Can you work these out from the model? Positions are in its coordinate system, mm. Face numbers are marked on the shaded views. A direction names the side the tool comes from. Round coordinates to 2 decimals unless told otherwise and drop trailing zeros. Write each loop counter-clockwise with the first axis right and the second up, starting at its lowest first coordinate (ties: lowest second). Pieces come first, ordered by that corner, then holes. Notation, with made-up numbers: M 54,73.25 L 62,73.25 A25 ccw 62,99.25 Z; hole C -9.75,22 d7. An arc over 180 degrees is marked long. Answer in a Markdown table with one row per item. Add a question column.
(1) Suppose I cut it at D-D, the plane z = 0.75. Write out the boundary of the cut face in (x, y).
(2) If I drill on probe 1 along X at (y, z) = (1, 5.5); probe 2 along Z at (x, y) = (-6, -5.75); probe 3 along Y at (x, z) = (-1.25, -2.5), over which ranges is the centre line in solid material (lowest first)?
(3) Suppose I cut it at A-A, the plane z = -5.5. Write out the boundary of the cut face in (x, y) (3 decimals), then the cut area to 3 significant figures.
(4) For the marked faces 1, 2 and 3, which set-ups out of +Z, -Z, +X, -X, +Y, -Y let a thin tool reach every point of the face, with its end or its side?
(5) I'm going to push flat-ended pins straight in: pin 1 (2.5 mm diameter, centred on x = -9, z = 5.5, fed in from +Y); pin 2 (1 mm diameter, centred on x = -4.5, y = -6.5, fed in from +Z); pin 3 (3 mm diameter, centred on x = 9, z = -5.5, fed in from -Y); pin 4 (0.9 mm diameter, centred on y = -2.5, z = -18, fed in from +X). Where does each tip first touch, or does it pass through?
(6) Suppose I cut it at B-B, the plane x = 9. Write out the boundary of the cut face in (y, z) (3 decimals).
(7) Suppose I cut it at C-C, the plane y = 1. Write out the boundary of the cut face in (x, z), then the cut area to 3 significant figures.
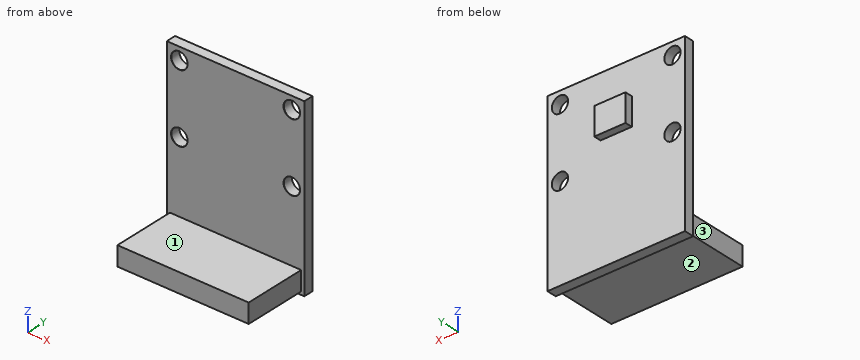
from build123d import *

# Parameters (mm, degrees)
SKETCH1_W                           = 22
SKETCH1_H                           = 28
BOSS_EXTRUDE1_DEPTH                 = 1.57
F_2_6_2_6_DIAMETER_HOLE1_AT_2_COUNT = 2
F_2_6_2_6_DIAMETER_HOLE1_AT_2_PITCH = 11
F_2_6_2_6_DIAMETER_HOLE1_AT_3_COUNT = 2
F_2_6_2_6_DIAMETER_HOLE1_AT_3_PITCH = 21.09502311
F_2_6_2_6_DIAMETER_HOLE1_AT_4_COUNT = 2
F_2_6_2_6_DIAMETER_HOLE1_AT_4_PITCH = 18
SKETCH5_W                           = 5
SKETCH5_H                           = 4.4
BOSS_EXTRUDE2_DEPTH                 = 1.2
SKETCH6_W                           = 21
SKETCH6_H                           = 3.08
BOSS_EXTRUDE3_DEPTH                 = 10


with BuildPart() as part:
    # Sketch1 → Boss-Extrude1 (new body)
    with BuildSketch(Plane(origin=(0, 0, 0), x_dir=(1, 0, 0), z_dir=(0, 1, 0))):
        with Locations((0, 6.5)):
            Rectangle(SKETCH1_W, SKETCH1_H)
    extrude(amount=BOSS_EXTRUDE1_DEPTH)

    # Sketch3 → Ø2.6 (2.6) Diameter Hole1 (revolve, cut)
    with BuildSketch(Plane(origin=(-9, 1.57, -5.5), x_dir=(0, 0, 1), z_dir=(1, 0, 0))):
        Polygon((0, 0), (0, 1.57), (1.325, 1.57), (1.3, 1.545), (1.3, 0), align=None)
    f_2_6_2_6_diameter_hole1 = revolve(axis=Axis((-9, 7.92, -5.5), (0, -1, 0)), mode=Mode.SUBTRACT)

    # Ø2.6 (2.6) Diameter Hole1 at 2: Ø2.6 (2.6) Diameter Hole1 ×2
    with Locations(*[(0, 0, i * F_2_6_2_6_DIAMETER_HOLE1_AT_2_PITCH) for i in range(1, F_2_6_2_6_DIAMETER_HOLE1_AT_2_COUNT)]):
        add(f_2_6_2_6_diameter_hole1, mode=Mode.SUBTRACT)

    # Ø2.6 (2.6) Diameter Hole1 at 3: Ø2.6 (2.6) Diameter Hole1 ×2
    with Locations(*[Vector(0.853281834, 0, 0.521450009) * (i * F_2_6_2_6_DIAMETER_HOLE1_AT_3_PITCH) for i in range(1, F_2_6_2_6_DIAMETER_HOLE1_AT_3_COUNT)]):
        add(f_2_6_2_6_diameter_hole1, mode=Mode.SUBTRACT)

    # Ø2.6 (2.6) Diameter Hole1 at 4: Ø2.6 (2.6) Diameter Hole1 ×2
    with Locations(*[(i * F_2_6_2_6_DIAMETER_HOLE1_AT_4_PITCH, 0, 0) for i in range(1, F_2_6_2_6_DIAMETER_HOLE1_AT_4_COUNT)]):
        add(f_2_6_2_6_diameter_hole1, mode=Mode.SUBTRACT)

    # Sketch5 → Boss-Extrude2 (add)
    with BuildSketch(Plane(origin=(0, 1.57, 0), x_dir=(1, 0, 0), z_dir=(0, 1, 0))):
        Rectangle(SKETCH5_W, SKETCH5_H)
    extrude(amount=BOSS_EXTRUDE2_DEPTH)

    # Sketch6 → Boss-Extrude3 (add)
    with BuildSketch(Plane(origin=(0, 0, 0), x_dir=(1, 0, 0), z_dir=(0, 1, 0))):
        with Locations((0, 18.46)):
            Rectangle(SKETCH6_W, SKETCH6_H)
    extrude(amount=-BOSS_EXTRUDE3_DEPTH)


solid = part.part
Calculated:
| question | item | result |
|---|---|---|
| 1 | outline | M -11,0 L 11,0 L 11,1.57 L 2.5,1.57 L 2.5,2.77 L -2.5,2.77 L -2.5,1.57 L -11,1.57 Z |
| 2 | probe 1 | -11 to -10.3, -7.7 to 7.7, 10.3 to 11 |
| 2 | probe 2 | -20 to -16.92 |
| 2 | probe 3 | 0 to 1.57 |
| 3 | outline | M -11,0 L -10.325,0 L -10.3,0.025 L -10.3,1.57 L -11,1.57 Z; M -7.7,0.025 L -7.675,0 L 7.675,0 L 7.7,0.025 L 7.7,1.57 L -7.7,1.57 Z; M 10.3,0.025 L 10.325,0 L 11,0 L 11,1.57 L 10.3,1.57 Z |
| 3 | area | 26.4 mm² |
| 4 | face 1 | +Z, +X, -X, -Y |
| 4 | face 2 | -Z, +X, -X, -Y |
| 4 | face 3 | +Z, -Z, -X, -Y |
| 5 | pin 1 | through |
| 5 | pin 2 | z = -16.92 |
| 5 | pin 3 | y = 0 |
| 5 | pin 4 | x = 10.5 |
| 6 | outline | M -10,-20 L 0,-20 L 0,-20.5 L 1.57,-20.5 L 1.57,-6.8 L 0.025,-6.8 L 0,-6.825 L 0,-16.92 L -10,-16.92 Z; M 0,-4.175 L 0.025,-4.2 L 1.57,-4.2 L 1.57,4.2 L 0.025,4.2 L 0,4.175 Z; M 0,6.825 L 0.025,6.8 L 1.57,6.8 L 1.57,7.5 L 0,7.5 Z |
| 7 | outline | M -11,-20.5 L 11,-20.5 L 11,7.5 L -11,7.5 Z; hole C -9,-5.5 d2.6; hole C -9,5.5 d2.6; hole C 9,-5.5 d2.6; hole C 9,5.5 d2.6 |
| 7 | area | 595 mm² |
